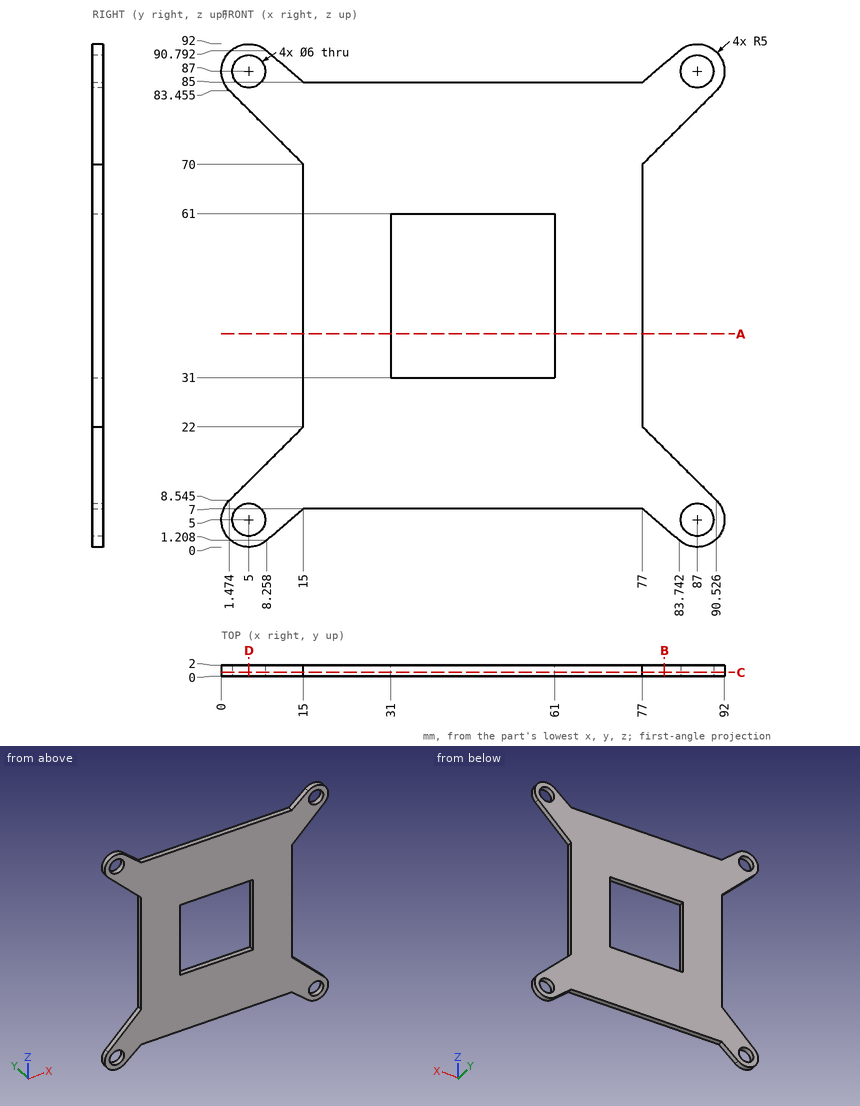
Design review of the part shown in the three views and the two pictorial views. Dimensions are in mm from the part's minimum x, y and z. Coordinates: 2 decimals unless noted, no trailing zeros. Loops run counter-clockwise (first coordinate to the right, second up) from the corner with the lowest first, then second, coordinate; pieces in that order, holes last. Notation, with made-up numbers: (58.25, -16.75) -> (65.25, -16.75) arc R17 cw to (65.25, 12.25) -> close; hole circle Ø10 at (71, 60.25). An arc over 180 degrees is marked (long way). Answer as CSV lines item,"result".
Item 1: Take a section at A-A, the plane z = 39. State the section outline as (x, y) points.
Results below:
outline,"(15, 0) -> (31, 0) -> (31, 2) -> (15, 2) -> close; (61, 0) -> (77, 0) -> (77, 2) -> (61, 2) -> close"
Item 2: Take a section at B-B, the plane x = 81. State the section outline as (y, z) points.
Results below:
outline,"(0, 3.56) -> (2, 3.56) -> (2, 18.02) -> (0, 18.02) -> close; (0, 73.98) -> (2, 73.98) -> (2, 88.44) -> (0, 88.44) -> close"
Item 3: Insertion check: pin 1 (0.6 mm diameter, centred on y = 1, z = 51, fed in from -X); pin 2 (0.6 mm diameter, centred on y = 0.5, z = 47.5, fed in from +X); pin 3 (0.6 mm diameter, centred on x = 38.5, y = 1, fed in from -Z). Each pin has a flat end and moves straight along its axis. Give the tip position at first contact, or say it passes through.
Results below:
pin 1,"stops at x = 15"
pin 2,"stops at x = 77"
pin 3,"stops at z = 7"
Item 4: Take a section at C-C, the plane y = 0.65. State the section outline as (x, z) points (1 decimal).
Results below:
outline,"(1.5, 8.5) arc R5 ccw to (8.3, 1.2) -> (15, 7) -> (77, 7) -> (83.7, 1.2) arc R5 ccw to (90.5, 8.5) -> (77, 22) -> (77, 70) -> (90.5, 83.5) arc R5 ccw to (83.7, 90.8) -> (77, 85) -> (15, 85) -> (8.3, 90.8) arc R5 ccw to (1.5, 83.5) -> (15, 70) -> (15, 22) -> close; hole circle Ø6 at (5, 5); hole circle Ø6 at (5, 87); hole (31, 31) -> (61, 31) -> (61, 61) -> (31, 61) -> close; hole circle Ø6 at (87, 5); hole circle Ø6 at (87, 87)"
Item 5: For L1, parallel to Z at x = 52, y = 0.15; L2, parallel to X at y = 1.6, z = 5.5 (1 decimal); L3, parallel to X at y = 0.55, z = 87 (1 decimal), list the stretches that pass through material, from the lowest coordinate up.
Results below:
L1,"z = 7 to 31, 61 to 85"
L2,"x = 0 to 2, 8 to 13.3, 78.7 to 84, 90 to 92"
L3,"x = 0 to 2, 8 to 12.7, 79.3 to 84, 90 to 92"
Item 6: Take a section at D-D, the plane x = 5. State the section outline as (y, z) points.
Results below:
outline,"(0, 0) -> (2, 0) -> (2, 2) -> (0, 2) -> close; (0, 8) -> (2, 8) -> (2, 12.05) -> (0, 12.05) -> close; (0, 79.95) -> (2, 79.95) -> (2, 84) -> (0, 84) -> close; (0, 90) -> (2, 90) -> (2, 92) -> (0, 92) -> close"
